```python
from build123d import *

# Parameters (mm, degrees)
SKETCH1_W           = 387.3
SKETCH1_H           = 409.62
BOSS_EXTRUDE1_DEPTH = 1.5875
SKETCH2_R           = 2.5
BOSS_EXTRUDE3_DEPTH = 100


with BuildPart() as part:
    # Sketch1 → Boss-Extrude1 (new body)
    with BuildSketch(Plane.XY):
        with Locations((0, -204.81)):
            Rectangle(SKETCH1_W, SKETCH1_H)
    extrude(amount=BOSS_EXTRUDE1_DEPTH)

    # Sketch2 → Boss-Extrude3 (add, symmetric)
    with BuildSketch(Plane(origin=(0, 0, 0), x_dir=(0, 0, -1), z_dir=(1, 0, 0))):
        with BuildLine():
            Line((-10.5875, 2), (-1.5875, -10))
            Line((-1.5875, -10), (-1.5875, 5))
            ThreePointArc((-1.5875, 5), (-8.16863883, 9.74341649), (-10.5875, 2))
        make_face()
        with Locations((-6.5875, 5)):
            Circle(SKETCH2_R, mode=Mode.SUBTRACT)
    extrude(amount=BOSS_EXTRUDE3_DEPTH, both=True)


solid = part.part
```
Here's how the part is built. I have some questions about the finished solid (model axes, mm). A direction names the side the tool comes from. Give positions to 0.01 mm unless a question says otherwise; leave off trailing zeros. Order: outer loops, then holes, each group sorted by start corner. A loop starts at its lowest first (then second) coordinate and runs counter-clockwise, first axis right, second up. Notation, with made-up numbers: (8, 89.25) -> (43, 89.25) arc R28 cw to (43, 125.25) -> close; hole circle Ø2 at (81, -19.5). An arc over 180 degrees is marked (long way). Use CSV: the item, a comma, the result in double quotes. Start each with the question number.
Item 1: On a 3-axis mill with a long thin cutter (end or side, diameter ignored), from which of +Z, -Z, +X, -X, +Y, -Y can I reach the whole of each face in a straight line? I mean faces 1 (the flat face through (-3, -202, 0)), 2 (the flat face through (-100, 2, 6)), 3 (the flat face through (100, 2, 6)). Say none if no direction works.
Item 2: Suppose I cut it at A-A (x = -21.5). List the corners of the cut face in (y, z) for me.
Item 3: Suppose I cut it at C-C (x = 138.5). List the corners of the cut face in (y, z) for me.
Item 4: If I drill on probe 1 along Z at (x, y) = (0.5, -151.5); probe 2 along Y at (x, z) = (-91.5, 7.25); probe 3 along Y at (x, z) = (-95.5, 6.5), over which ranges is the centre line in solid material (lowest first)? Write a range as [from, to].
Item 5: I'm going to push flat-ended pins straight in: P1, Ø5, axis at y = -2, z = 5, coming from the +X side; P2, Ø5, axis at y = -3.5, z = 9, coming from the -X side; P3, Ø2, axis at x = -91, z = 9, coming from the +Y side; P4, Ø4.5, axis at y = 5, z = 6.59, coming from the +X side. Where does each tip first touch, or does it pass through?
Item 6: Suppose I cut it at B-B (y = -294.5). List the corners of the cut face in (x, z) for me, and give its area (3 significant figures).
Answer block:
1,face 1,"-Z, +X, -X, +Y, -Y"
1,face 2,"+Z, -X, +Y, -Y"
1,face 3,"+Z, +X, +Y, -Y"
2,outline,"(-409.62, 0) -> (0, 0) -> (0, 1.59) -> (5, 1.59) arc R5 ccw (long way) to (2, 10.59) -> (-10, 1.59) -> (-409.62, 1.59) -> close; hole circle Ø5 at (5, 6.59)"
3,outline,"(-409.62, 0) -> (0, 0) -> (0, 1.59) -> (-409.62, 1.59) -> close"
4,probe 1,"z = [0, 1.59]"
4,probe 2,"y = [-2.45, 2.59], [7.41, 9.96]"
4,probe 3,"y = [-3.45, 2.5], [7.5, 10]"
5,P1,"stops at x = 100"
5,P2,"stops at x = -100"
5,P3,"stops at y = 9.8"
5,P4,"passes through"
6,outline,"(-193.65, 0) -> (193.65, 0) -> (193.65, 1.59) -> (-193.65, 1.59) -> close"
6,area,"615 mm^2"
